from build123d import *

# Parameters (mm, degrees)
ESQUISSE28_R             = 6.5
ENL_V_MAT_EXTRU_16_DEPTH = 76.4917214
CONG_1_R                 = 10
ESQUISSE29_R             = 4
BOSS_EXTRU_1_DEPTH       = 6
ESQUISSE30_R             = 19.501187477
ESQUISSE30_R_2           = 15
BOSS_EXTRU_2_DEPTH       = 9.735855
CONG_2_R                 = 10


with BuildPart() as part:
    # Esquisse27 → Révolution1 (revolve)
    with BuildSketch(Plane(origin=(0, 0, 0), x_dir=(0, 0, -1), z_dir=(1, 0, 0)), mode=Mode.PRIVATE) as r_volution1_sk:
        Polygon((8, 14.29), (8, 0), (57, 0), (57, 14.29), (65, 14.29), (65, 35), (55, 35), (55, 19.501187477), (64.735853824, 19.501187477), (64.735853824, 15), (10, 15), (10, 35), (0, 35), (0, 14.29), align=None)
    revolve(r_volution1_sk.sketch.rotate(Axis((0, 0, -10), (0, 0, -1)), 90), axis=Axis((0, 0, -10), (0, 0, -1)))

    # Esquisse28 → Enlèv. mat.-Extru.16 (cut, through all)
    with BuildSketch(Plane(origin=(0, 0, -57), x_dir=(-1, 0, 0), z_dir=(0, 0, -1))):
        Circle(ESQUISSE28_R)
    extrude(amount=-ENL_V_MAT_EXTRU_16_DEPTH, mode=Mode.SUBTRACT)

    # Congé1
    cong_1_edges = [part.edges().sort_by_distance(p)[0] for p in [
        (-15, 0, -10),
    ]]
    fillet(cong_1_edges, radius=CONG_1_R)

    # Esquisse29 → Boss.-Extru.1 (add)
    with BuildSketch(Plane(origin=(0, 0, -65), x_dir=(-1, 0, 0), z_dir=(0, 0, -1))):
        with Locations(Location((0, 25, 0), (0, 0, 180))):
            Circle(ESQUISSE29_R)
        with Locations(Location((25, 0, 0), (0, 0, 180))):
            Circle(ESQUISSE29_R)
        with Locations(Location((0, -25, 0), (0, 0, 180))):
            Circle(ESQUISSE29_R)
        with Locations(Location((-25, 0, 0), (0, 0, 180))):
            Circle(ESQUISSE29_R)
    extrude(amount=BOSS_EXTRU_1_DEPTH)

    # Esquisse30 → Boss.-Extru.2 (add)
    with BuildSketch(Plane.XY.offset(-64.735853824)):
        Circle(ESQUISSE30_R)
        Circle(ESQUISSE30_R_2, mode=Mode.SUBTRACT)
    extrude(amount=BOSS_EXTRU_2_DEPTH)

    # Congé2
    # the kernel refuses this fillet: 10 mm, written as the material it adds along each edge
    with BuildSketch(Plane(origin=(0, 0, -54.999998824), x_dir=(1, 0, 0), z_dir=(0, -1, 0))) as cong_2_piece_1:
        with BuildLine():
            CenterArc((15 + CONG_2_R, CONG_2_R), CONG_2_R, 180, 90)
            Line((15 + CONG_2_R, 0), (15 + CONG_2_R, -CONG_2_R * 0.02))
            Line((15 + CONG_2_R, -CONG_2_R * 0.02), (15 - CONG_2_R * 0.02, -CONG_2_R * 0.02))
            Line((15 - CONG_2_R * 0.02, -CONG_2_R * 0.02), (15 - CONG_2_R * 0.02, CONG_2_R))
            Line((15 - CONG_2_R * 0.02, CONG_2_R), (15, CONG_2_R))
        make_face()
    revolve(axis=Axis((0, 0, -54.999998824), (0, 0, 1)))


solid = part.part
Model file for the job. Use its own axes, mm. A direction names the side the tool comes from. Round coordinates to 2 decimals unless told otherwise and drop trailing zeros. Loops run counter-clockwise (first coordinate to the right, second up) from the corner with the lowest first, then second, coordinate; pieces in that order, holes last. Notation, with made-up numbers: (-24.75, 55) -> (33.25, 55) arc R17 ccw to (33.25, 71) -> close; hole circle Ø10 at (32, 55). An arc over 180 degrees is marked (long way). Answer as CSV lines item,"result". Start each with the question number.
1) Pin check, flat tips, straight feed: P1, Ø14.5, axis at x = 4, y = 1.5, coming from the -Z side; P2, Ø1.5, axis at x = -8.5, z = -9, coming from the +Y side; P3, Ø6, axis at x = -14.5, z = -44, coming from the +Y side; P4, Ø4, axis at x = -24.5, z = -51.5, coming from the +Y side. Stop position of each tip, or through.
2) Mould opens along Z. For faces 5 (the face through (0, 25, -71)), 6 (the face through (-24, -8, -55)), 7 (the face through (-0.521, 21.034, -67.958)), 8 (the face through (24, -8, -10)) say: +Z half, -Z half, draft (parallel to the pull), parting line (faces both ways), or undercut.
3) Slice it at C-C (z = -18.5). List the corners of the cut face in (x, y), plus the area to 3 significant figures.
4) Probe line 1 along Z through (x, y) = (-26.5, 7.5); line 2 along Y through (x, z) = (0, -45.5); line 3 along Y through (x, z) = (0, -62). List the from-to ranges inside material, lowest first.
5) Slice it at B-B (z = -44). List the corners of the cut face in (x, y), plus the area to 3 significant figures.
6) Slice it at A-A (y = 26.5). List the corners of the cut face in (x, z), plus the area to 3 significant figures.
7) Tool access for faces 1 (the face through (0, -25, -71)), 2 (the face through (21.8, 2.4, -68)), 3 (the face through (8.06, -12.65, -32.32)), 4 (the face through (6, 3, -8)): list every direction of +Z, -Z, +X, -X, +Y, -Y with a clear straight run to the whole face (end or side of a thin tool).
Filled in:
1,P1,"stops at z = -57"
1,P2,"stops at y = 34.13"
1,P3,"stops at y = 9.63"
1,P4,"passes through"
2,face 5,"-Z half"
2,face 6,"undercut"
2,face 7,"draft"
2,face 8,"undercut"
3,outline,"circle Ø30.23 at (0, 0); hole circle Ø13 at (0, 0)"
3,area,"585 mm2"
4,line 1,"z = -65 to -55, -10 to 0"
4,line 2,"y = -15.01 to -6.5, 6.5 to 15.01"
4,line 3,"y = -35 to -14.29, 14.29 to 35"
5,outline,"circle Ø30 at (0, 0); hole circle Ø13 at (0, 0)"
5,area,"574 mm2"
6,outline,"(-22.86, -65) -> (-3.71, -65) -> (-3.71, -71) -> (3.71, -71) -> (3.71, -65) -> (22.86, -65) -> (22.86, -55) -> (-22.86, -55) -> close; (-22.86, -10) -> (22.86, -10) -> (22.86, 0) -> (-22.86, 0) -> close"
6,area,"959 mm2"
7,face 1,"-Z, +X, -X, +Y, -Y"
7,face 2,"-Z"
7,face 3,"none"
7,face 4,"+Z"
